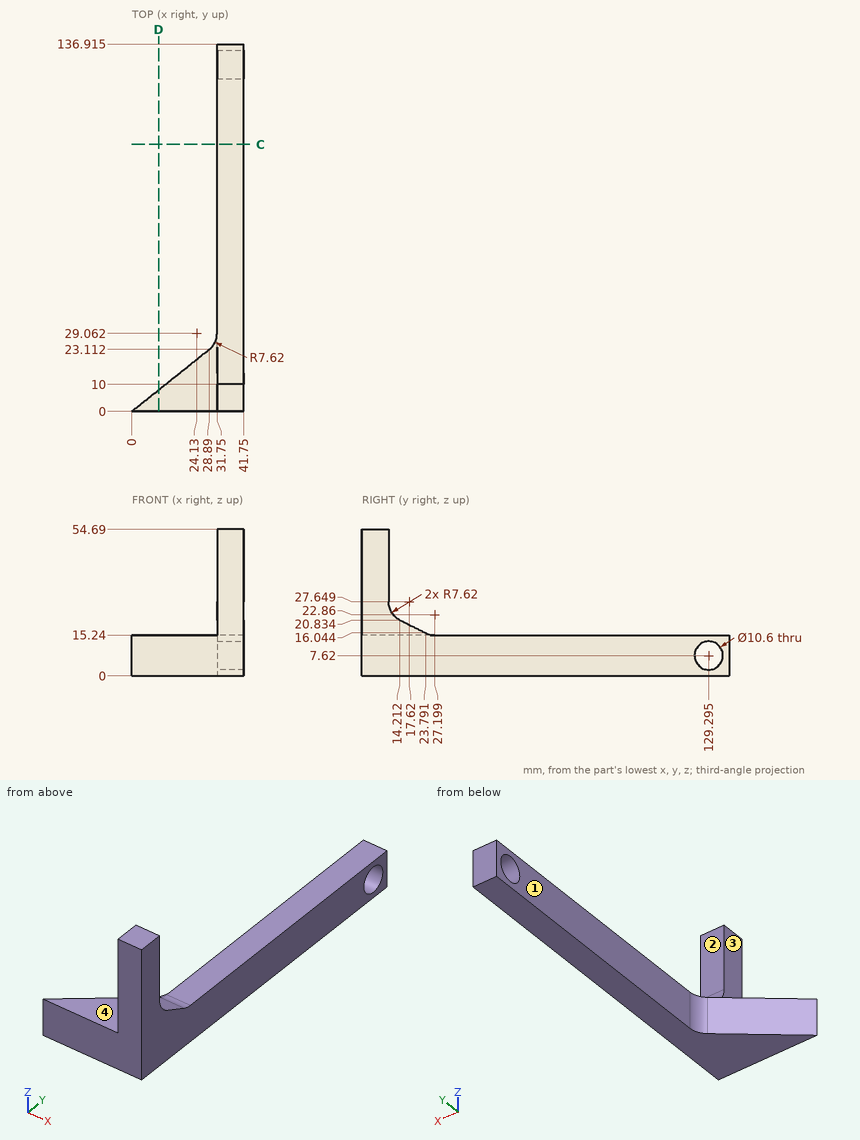
For this review, use the dimensioned drawing (mm, ordinates from the lowest corner) and the shaded views. A direction names the side the tool comes from. Coordinates: 2 decimals unless noted, no trailing zeros. Order: outer loops, then holes, each group sorted by start corner. A loop starts at its lowest first (then second) coordinate and runs counter-clockwise, first axis right, second up. Notation, with made-up numbers: (88, 8.5) - (105, 8.5) arc R25 ccw to (105, 27.5) - close; hole circle Ø3 at (80.25, -4.75). An arc over 180 degrees is marked (long way). Answer in a Markdown table with one row per item.
(1) Wall thickness on line 1 along Y through (x, z) = (35.5, 7.62) (1 decimal); line 2 along X through (y, z) = (80.5, 4): over which ranges is each line inside the solid? List them lowest first. Write a range as from..to.
Checked values:
| item | result |
|---|---|
| line 1 | 0..124, 134.6..136.9 |
| line 2 | 31.75..41.75 |
(2) For the marked faces 1, 2, 3 and 4, list the 3-axis set-ups (+Z, -Z, +X, -X, +Y, -Y) from which the entire face can be reached by the end or side of a thin tool; tool diameter is ignored.
Checked values:
| item | result |
|---|---|
| face 1 | +Z, -Z, -X, +Y |
| face 2 | +Z, +X, -X, +Y |
| face 3 | +Z, -X, +Y, -Y |
| face 4 | +Z, -X, +Y |
(3) Consider section D-D on x = 10. State the section outline as (y, z) points, plus the area to 3 significant figures.
Checked values:
| item | result |
|---|---|
| outline | (0, 0) - (8, 0) - (8, 15.24) - (0, 15.24) - close |
| area | 122 mm^2 |
(4) Consider section C-C on y = 99.5. State the section outline as (x, z) points, plus the area to 3 significant figures.
Checked values:
| item | result |
|---|---|
| outline | (31.75, 0) - (41.75, 0) - (41.75, 15.24) - (31.75, 15.24) - close |
| area | 152 mm^2 |
(5) Clearance check with flat-ended pins moving along their axes: pin 1 (2 mm diameter, centred on y = 31, z = 11.5, fed in from -X); pin 2 (11 mm diameter, centred on x = 35, z = 44, fed in from +Y); pin 3 (12.5 mm diameter, centred on x = 21, y = 66, fed in from +Z). State where each tip first meets the part, or that it passes through.
Checked values:
| item | result |
|---|---|
| pin 1 | x = 31.75 |
| pin 2 | y = 10 |
| pin 3 | through |
